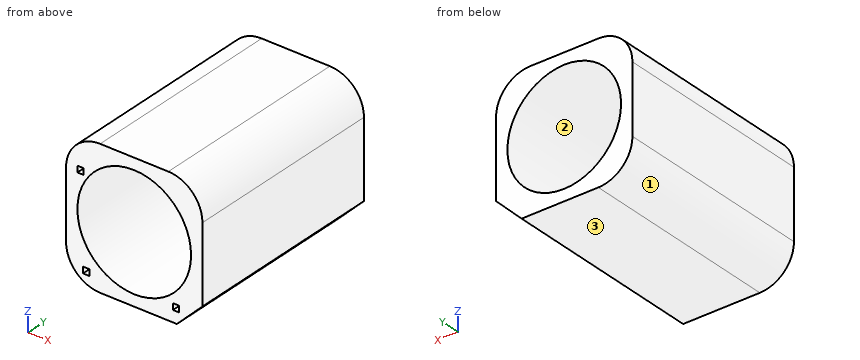
from build123d import *

# Parameters (mm, degrees)
SKETCH1_R           = 2.5
BOSS_EXTRUDE1_DEPTH = 4.5
SKETCH2_W           = 0.275
SKETCH2_H           = 0.275
CUT_EXTRUDE1_DEPTH  = 1


with BuildPart() as part:
    # Sketch1 → Boss-Extrude1 (new body, symmetric)
    with BuildSketch(Plane(origin=(0, 0, 0), x_dir=(1, 0, 0), z_dir=(0, 1, 0))):
        with BuildLine():
            Line((3, 1.875), (1.875, 3))
            Line((1.875, 3), (-1.5, 3))
            ThreePointArc((-1.5, 3), (-2.560660172, 2.560660172), (-3, 1.5))
            Line((-3, 1.5), (-3, -1.5))
            ThreePointArc((-3, -1.5), (-2.560660172, -2.560660172), (-1.5, -3))
            Line((-1.5, -3), (1.5, -3))
            ThreePointArc((1.5, -3), (2.560660172, -2.560660172), (3, -1.5))
            Line((3, -1.5), (3, 1.875))
        make_face()
        Circle(SKETCH1_R, mode=Mode.SUBTRACT)
    extrude(amount=BOSS_EXTRUDE1_DEPTH, both=True)

    # Sketch2 → Cut-Extrude1 (cut)
    with BuildSketch(Plane.XZ.offset(4.5)):
        with Locations((-2.3625, 1.6125)):
            Rectangle(SKETCH2_W, SKETCH2_H)
        with Locations((-2.1125, -2.3625)):
            Rectangle(SKETCH2_W, SKETCH2_H)
        with Locations((1.8425, -2.3625)):
            Rectangle(SKETCH2_W, SKETCH2_H)
    extrude(amount=-CUT_EXTRUDE1_DEPTH, mode=Mode.SUBTRACT)


solid = part.part
Geometry: final body of the model. Coordinates: model frame, mm. Face numbers are marked on the shaded views. Round coordinates to 2 decimals unless told otherwise and drop trailing zeros. Loops run counter-clockwise (first coordinate to the right, second up) from the corner with the lowest first, then second, coordinate; pieces in that order, holes last. Notation, with made-up numbers: M 29.5,56.25 L 55.5,56.25 A14 cw 55.5,66.25 Z; hole C 33.5,10.5 d5. An arc over 180 degrees is marked long. One line per question, with ' | ' between items.
(1) Pull-direction query (X, two-part tool) for the marked faces 1, 2 and 3; classes: +X half, -X half, draft (parallel to the pull), parting line (faces both ways), or undercut.
Check result:
face 1: -X half | face 2: undercut | face 3: draft
(2) Cut plane A-A on x = 0. Return the cut outline in (y, z).
Check result:
outline: M -4.5,-3 L 4.5,-3 L 4.5,-2.5 L -4.5,-2.5 Z; M -4.5,2.5 L 4.5,2.5 L 4.5,3 L -4.5,3 Z
(3) Material intervals for line 1 along Z through (x, y) = (0, -2.5); line 2 along Z through (x, y) = (0.95, 0.75), sorted ascending. Write a range as from..to.
Check result:
line 1: z = -3..-2.5, 2.5..3 | line 2: z = -3..-2.31, 2.31..3
(4) Cut plane C-C on y = -3. Return the cut outline in (x, z) (3 decimals).
Check result:
outline: M -3,-1.5 A1.5 ccw -1.5,-3 L 1.875,-3 L 3,-1.875 L 3,1.5 A1.5 ccw 1.5,3 L -1.5,3 A1.5 ccw -3,1.5 Z; hole C 0,0 d5
(5) Cut plane B-B on z = 0. Return the cut outline in (x, y), plus the area to 3 significant figures.
Check result:
outline: M -3,-4.5 L -2.5,-4.5 L -2.5,4.5 L -3,4.5 Z; M 2.5,-4.5 L 3,-4.5 L 3,4.5 L 2.5,4.5 Z | area: 9.00 mm2
(6) Cut plane D-D on z = 2.65. Return the cut outline in (x, y), plus the area to 3 significant figures.
Check result:
outline: M -2.46,-4.5 L 2.46,-4.5 L 2.46,4.5 L -2.46,4.5 Z | area: 44.3 mm2
